from build123d import *

# Parameters (mm, degrees)
F0_W     = 80
F0_H     = 45
F0_R     = 5.5
F1_DEPTH = 50
F3_DEPTH = 39
F4_DEPTH = 45


with BuildPart() as f1:
    # F0 (on Top) → F1 (new body)
    with BuildSketch(Plane.XY):
        Rectangle(F0_W, F0_H)
        with Locations((-31.096611172, 0)):
            Circle(F0_R, mode=Mode.SUBTRACT)
        with Locations((31.096611172, 0)):
            Circle(F0_R, mode=Mode.SUBTRACT)
    extrude(amount=F1_DEPTH)

    # F2 (on Front) → F3 (join, symmetric)
    with BuildSketch(Plane.XZ):
        with BuildLine():
            ThreePointArc((-20, 50), (0, 30), (20, 50))
            Line((20, 50), (13, 50))
            ThreePointArc((13, 50), (0, 37), (-13, 50))
            Line((-13, 50), (-20, 50))
        make_face()
    extrude(amount=F3_DEPTH, both=True)

    # F4 (cut, through all): a face of the model
    f4_faces = [f1.faces().sort_by_distance(p)[0] for p in [
        (0, -22.5, 44.4826286395),
    ]]
    extrude(f4_faces, amount=-F4_DEPTH, mode=Mode.SUBTRACT)


solid = f1.part
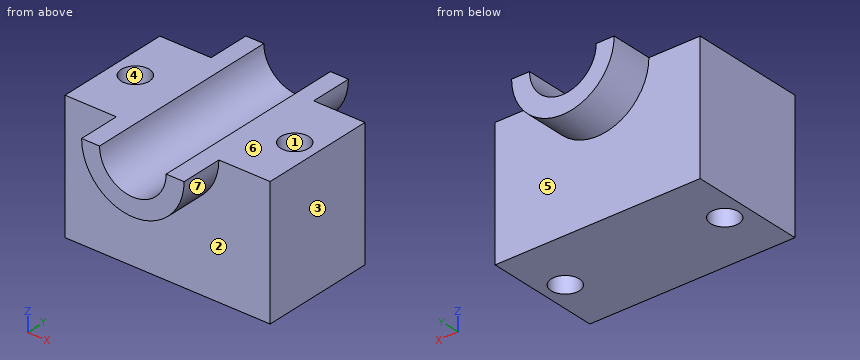
The model under review builds one solid part; all positions refer to its coordinate system, in mm. Face numbers are marked on the shaded views. A direction names the side the tool comes from. Round coordinates to 2 decimals unless told otherwise and drop trailing zeros. Loops run counter-clockwise (first coordinate to the right, second up) from the corner with the lowest first, then second, coordinate; pieces in that order, holes last. Notation, with made-up numbers: (-5, 28.5) -> (9, 28.5) arc R20 ccw to (9, 57.5) -> close; hole circle Ø3 at (54.5, 2). An arc over 180 degrees is marked (long way). One line per question, with ' | ' between items. Start each with the question number.
Item 1: Add section B-B, the plane y = 0. Write out the cut boundary in (x, z), then the cut area to 3 significant figures.
Item 2: Add section A-A, the plane x = -31.5. Write out the cut boundary in (y, z), then the cut area to 3 significant figures.
Item 3: Machinability: for the marked faces 5, 6 and 7, which of the approach directions +Z, -Z, +X, -X, +Y, -Y give a long, thin tool a straight path to every point of the face, cutting with its end or side? Answer none if there is none.
Item 4: Draft analysis for pull direction Y (two halves, no side actions). For the marked faces 1, 2, 3 and 4, state which applies: +Y half, -Y half, draft (parallel to the pull), parting line (faces both ways), or undercut.
Item 5: Add section C-C, the plane z = 46.5. Write out the cut boundary in (x, y).
Item 6: For pin 1 (6 mm diameter, centred on x = -29.5, y = -20.5, fed in from -Z); pin 2 (1.5 mm diameter, centred on x = 23, z = 37.5, fed in from -Y); pin 3 (1.5 mm diameter, centred on x = 12, y = -24, fed in from -Z), all flat-tipped, find the tip position at first contact; note any pin that passes through.
Item 7: Add section D-D, the plane z = 10.5. Write out the cut boundary in (x, y), then the cut area to 3 significant figures.
Item 8: Wall thickness on line 1 along X through (y, z) = (4, 16.5); line 2 along X through (y, z) = (-1, 30); line 3 along Y through (x, z) = (-22.5, 30): over which ranges is each line inside the solid? List them lowest first. Write a range as [from, to].
Return value:
1) outline: (-40, 0) -> (-36.6, 0) -> (-36.6, 50) -> (-40, 50) -> close; (-25.6, 0) -> (25.6, 0) -> (25.6, 50) -> (13, 50) arc R13 cw to (-13, 50) -> (-25.6, 50) -> close; (36.6, 0) -> (40, 0) -> (40, 50) -> (36.6, 50) -> close | area: 2,630 mm2
2) outline: (-22.5, 0) -> (-5.49, 0) -> (-5.49, 50) -> (-22.5, 50) -> close; (5.49, 0) -> (22.5, 0) -> (22.5, 50) -> (5.49, 50) -> close | area: 1,700 mm2
3) face 5: -Z, +Y | face 6: +Z, +X, -X, +Y, -Y | face 7: -Z, -Y
4) face 1: undercut | face 2: -Y half | face 3: draft | face 4: undercut
5) outline: (-40, -22.5) -> (-19.69, -22.5) -> (-19.69, -39) -> (-12.52, -39) -> (-12.52, 39) -> (-19.69, 39) -> (-19.69, 22.5) -> (-40, 22.5) -> close; (12.52, -39) -> (19.69, -39) -> (19.69, -22.5) -> (40, -22.5) -> (40, 22.5) -> (19.69, 22.5) -> (19.69, 39) -> (12.52, 39) -> close; hole circle Ø11 at (-31.1, 0); hole circle Ø11 at (31.1, 0)
6) pin 1: stops at z = 0 | pin 2: stops at y = -22.5 | pin 3: stops at z = 33.46
7) outline: (-40, -22.5) -> (40, -22.5) -> (40, 22.5) -> (-40, 22.5) -> close; hole circle Ø11 at (-31.1, 0); hole circle Ø11 at (31.1, 0) | area: 3,410 mm2
8) line 1: x = [-40, -34.87], [-27.32, 27.32], [34.87, 40] | line 2: x = [-40, -36.5], [-25.69, 25.69], [36.5, 40] | line 3: y = [-22.5, 22.5]
